The listing builds one solid part. Answer for the finished solid, in the listing's coordinates (mm). Face numbers are marked on the shaded views. A direction names the side the tool comes from. Coordinates: 2 decimals unless noted, no trailing zeros. Loops run counter-clockwise (first coordinate to the right, second up) from the corner with the lowest first, then second, coordinate; pieces in that order, holes last. Notation, with made-up numbers: (52.5, 11.5) -> (87.5, 11.5) arc R30 ccw to (87.5, 39.5) -> close; hole circle Ø8 at (20, 15). An arc over 180 degrees is marked (long way). Answer in a Markdown table with one row per item.
Autodesk Inventor part; units mm, degrees
ref_plane "YZ Plane" through (0, 0, 0) normal (1, 0, 0) x (0, 1, 0)
ref_plane "XZ Plane" through (0, 0, 0) normal (0, 1, 0) x (-1, 0, 0)
ref_plane "XY Plane" through (0, 0, 0) normal (0, 0, 1) x (1, 0, 0)
sketch "Sketch1" plane through (0, 0, 0) normal (0, 1, 0) x (-1, 0, 0)
  circle A0 centre (0, 0) radius 32.5
  arc A1 (2, 1.5) -> (2, -1.5) centre (0, 0) ccw
  line L0 (-2.5, 0) -> (2, 0) construction
  line L1 (2, 0) -> (2, 1.5)
  line L2 (2, -1.5) -> (2, 0)
  dimension "d0" = 65
extrude "Extrusion1" add sketch "Sketch1" along normal blind 5
sketch "Sketch2" plane through (0, 5, 0) normal (0, 1, 0) x (1, 0, 0)
  circle A0 centre (0, 0) radius 5
  arc A1 (-2, -1.5) -> (-2, 1.5) centre (0, 0) ccw
  arc A2 (-2, -1.5) -> (-2, 1.5) centre (0, 0) ccw
  line L0 (-2, -1.5) -> (-2, 1.5)
  line L1 (-2, -1.5) -> (-2, 1.5)
  dimension "d6" = 10
extrude "Extrusion2" add sketch "Sketch2" along normal blind 10
properties part number "kolo"
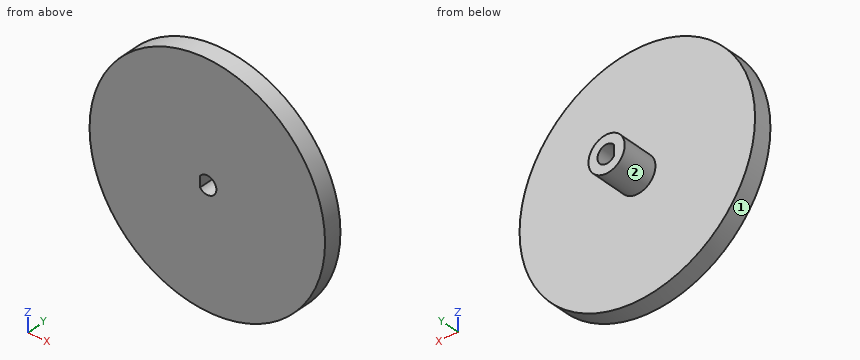
Item 1: Find the intervals of material crossed by probe 1 along Z at (x, y) = (0, 8); probe 2 along Z at (x, y) = (0, 3.5); probe 3 along Y at (x, z) = (-22, 15), in increasing order.
Findings below:
| item | result |
|---|---|
| probe 1 | z = -5 to -2.5, 2.5 to 5 |
| probe 2 | z = -32.5 to -2.5, 2.5 to 32.5 |
| probe 3 | y = 0 to 5 |
Item 2: A cutting plane is placed at A-A, the plane z = 0. Determine the outline of the cut face in (x, y).
Findings below:
| item | result |
|---|---|
| outline | (-32.5, 0) -> (-2, 0) -> (-2, 15) -> (-5, 15) -> (-5, 5) -> (-32.5, 5) -> close; (2.5, 0) -> (32.5, 0) -> (32.5, 5) -> (5, 5) -> (5, 15) -> (2.5, 15) -> close |
Item 3: Flat-ended cylindrical pins translate along their axes: pin 1 Ø2.5 at (y, z) = (7.5, -0.5) entering from +X; pin 2 Ø6 at (x, z) = (18, 7) entering from +Y; pin 3 Ø6 at (x, y) = (-12.5, 3.5) entering from -Z. Find the tip coordinate at first contact, or state that the pin passes through.
Findings below:
| item | result |
|---|---|
| pin 1 | stops at x = 5 |
| pin 2 | stops at y = 5 |
| pin 3 | stops at z = -31.08 |
Item 4: A cutting plane is placed at C-C, the plane y = 3. Determine the outline of the cut face in (x, z).
Findings below:
| item | result |
|---|---|
| outline | circle Ø65 at (0, 0); hole (-2, -1.5) arc R2.5 ccw (long way) to (-2, 1.5) -> close |
Item 5: A tool of negligible diameter and unlimited length cuts with its end or side. For the marked faces 1 and 2, from which of +Z, -Z, +X, -X, +Y, -Y can it reach the whole face along a straight path? Write none if from no direction.
Findings below:
| item | result |
|---|---|
| face 1 | +Y, -Y |
| face 2 | +Y |
Item 6: A cutting plane is placed at B-B, the plane x = 0. Determine the outline of the cut face in (y, z), plus the area to 3 significant figures.
Findings below:
| item | result |
|---|---|
| outline | (0, -32.5) -> (5, -32.5) -> (5, -5) -> (15, -5) -> (15, -2.5) -> (0, -2.5) -> close; (0, 2.5) -> (15, 2.5) -> (15, 5) -> (5, 5) -> (5, 32.5) -> (0, 32.5) -> close |
| area | 350 mm2 |
Item 7: A cutting plane is placed at D-D, the plane x = -8. Determine the outline of the cut face in (y, z), plus the area to 3 significant figures.
Findings below:
| item | result |
|---|---|
| outline | (0, -31.5) -> (5, -31.5) -> (5, 31.5) -> (0, 31.5) -> close |
| area | 315 mm2 |
